Job drawing, mm, ordinate dimensions from the low corner. One solid piece. A direction names the side the tool comes from. Round coordinates to 2 decimals unless told otherwise and drop trailing zeros. Loops run counter-clockwise (first coordinate to the right, second up) from the corner with the lowest first, then second, coordinate; pieces in that order, holes last. Notation, with made-up numbers: M 27.25,2 L 32.25,2 A28 cw 32.25,30 Z; hole C -12,63.5 d1. An arc over 180 degrees is marked long. Use a Markdown table: item, result. Add a question column.
(1) Flat gauge pins, fed straight in: P1, Ø11.5, axis at x = 22.5, y = 19.5, coming from the +Z side; P2, Ø1.5, axis at y = 27, z = 3, coming from the -X side; P3, Ø8, axis at x = 16.5, z = 4.5, coming from the -Y side. Where does each tip first touch, or does it go through?
(2) Band-saw the part on A-A, the plane x = 18.5. Write the cut outline in (y, z).
(3) Which spindle directions (+Z, -Z, +X, -X, +Y, -Y) get a long thin tool onto all of the face, cutting with end or side? Do the marked faces 1, 2, 3, 4 and 5. Say none if no direction does.
(4) Band-saw the part on D-D, the plane x = 23. Write the cut outline in (y, z).
(5) Band-saw the part on B-B, the plane y = 3.75. Write the cut outline in (x, z).
(6) Wall check: L1, parallel to Y at x = 24.25, z = 9.5; L2, parallel to X at y = 19, z = 7.5; L3, parallel to Y at x = 3.5, z = 17.75. Give the ranges that are in metal, low to high.
(7) Band-saw the part on C-C, the plane z = 6. Write the cut outline in (x, y), and give its area (3 significant figures).
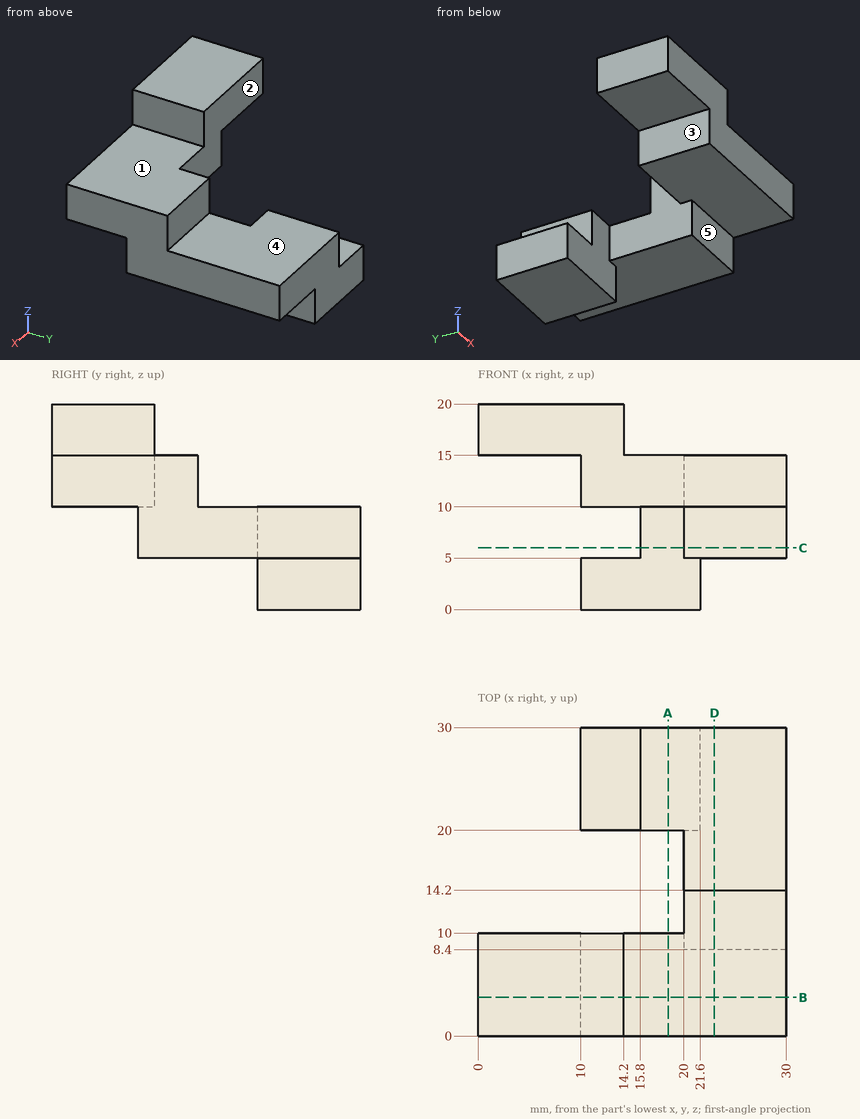
Return value:
| question | item | result |
|---|---|---|
| 1 | P1 | z = 15 |
| 1 | P2 | x = 10 |
| 1 | P3 | y = 8.4 |
| 2 | outline | M 0,10 L 10,10 L 10,15 L 0,15 Z; M 20,0 L 30,0 L 30,10 L 20,10 Z |
| 3 | face 1 | +Z, +X, +Y, -Y |
| 3 | face 2 | +Z, -Z, -X, +Y |
| 3 | face 3 | -Z, -X, +Y, -Y |
| 3 | face 4 | +Z, +X, -X, +Y |
| 3 | face 5 | -Z, +X, -X, -Y |
| 4 | outline | M 0,10 L 8.4,10 L 8.4,5 L 30,5 L 30,10 L 14.2,10 L 14.2,15 L 0,15 Z |
| 5 | outline | M 0,15 L 10,15 L 10,10 L 30,10 L 30,15 L 14.2,15 L 14.2,20 L 0,20 Z |
| 6 | L1 | 8.4 to 30 |
| 6 | L2 | 20 to 30 |
| 6 | L3 | 0 to 10 |
| 7 | outline | M 15.8,20 L 20,20 L 20,8.4 L 30,8.4 L 30,30 L 15.8,30 Z |
| 7 | area | 258 mm^2 |
